Source: three-view drawing plus pictorial views. Frame: mm from the lowest corner of the part. A direction names the side the tool comes from. Coordinates: 2 decimals unless noted, no trailing zeros. Write each loop counter-clockwise with the first axis right and the second up, starting at its lowest first coordinate (ties: lowest second). Pieces come first, ordered by that corner, then holes. Notation, with made-up numbers: (-27.5, -40) - (14.5, -40) arc R23 cw to (14.5, -13) - close; hole circle Ø2 at (10.5, 68.25). An arc over 180 degrees is marked (long way). One line per item, written item: value.
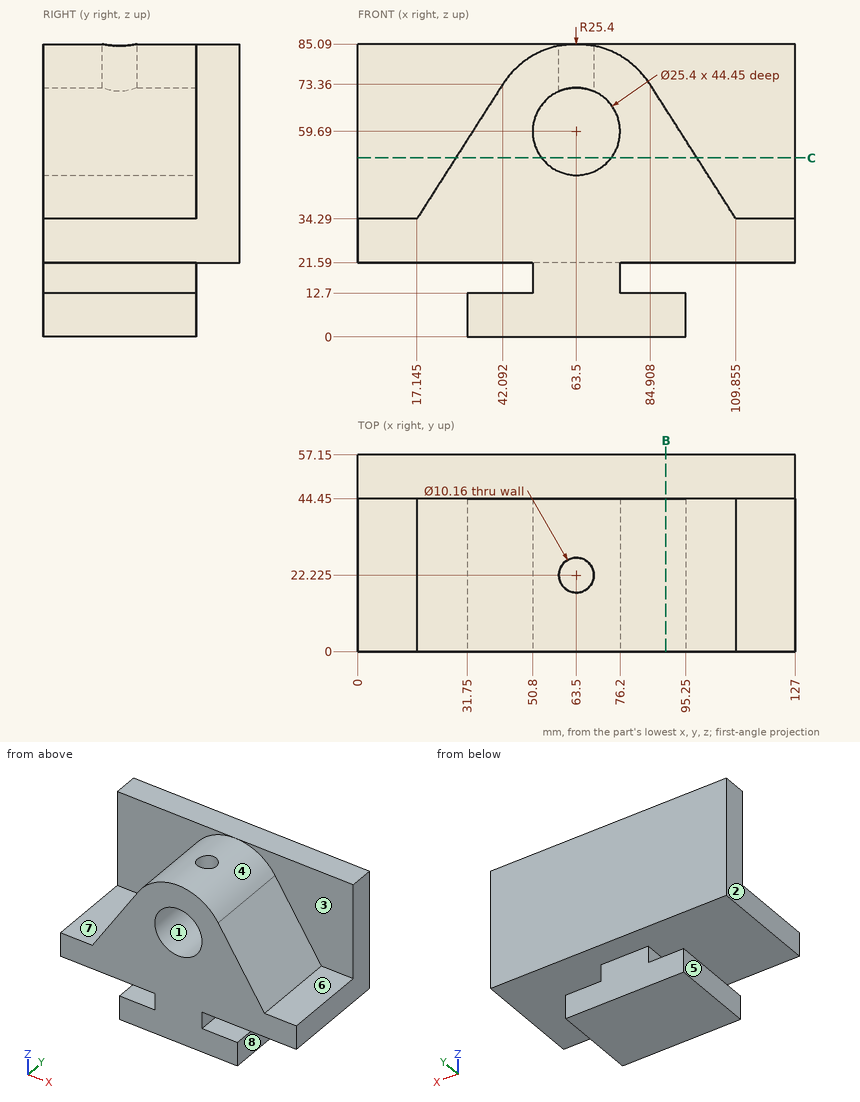
1) Section query C-C on z = 52. Output: boundary loops of the cut face in (x, y), then the cut area to 3 significant figures.
Values found:
outline: (0, 44.45) - (28.45, 44.45) - (28.45, 0) - (53.39, 0) - (53.39, 44.45) - (73.61, 44.45) - (73.61, 0) - (98.55, 0) - (98.55, 44.45) - (127, 44.45) - (127, 57.15) - (0, 57.15) - close
area: 3,830 mm2
2) Material intervals for line 1 (Z direction, x = 63.5, y = 10); line 2 (Z direction, x = 9.5, y = 5); line 3 (Y direction, x = 55, z = 19), sorted ascending.
Values found:
line 1: 0 to 46.99, 72.39 to 85.09
line 2: 21.59 to 34.29
line 3: 0 to 44.45
3) Contact query for flat-ended pins moving along their axis: P1, Ø19, axis at x = 12, y = 27, coming from the +Z side; P2, Ø7, axis at y = 27, z = 17.5, coming from the +X side; P3, Ø12.5, axis at x = 64.5, z = 60, coming from the -Y side. Output: stop coordinate, or through.
Values found:
P1: z = 41.11
P2: x = 76.2
P3: y = 44.45
4) Reachability of the marked faces 4, 5, 6, 7 and 8 from +Z, -Z, +X, -X, +Y, -Y: full face, straight path, thin tool, end or side. Return the list, or none.
Values found:
face 4: +Z, -Y
face 5: -Z, -X, +Y, -Y
face 6: +Z, +X, -Y
face 7: +Z, -X, -Y
face 8: -Z, +X, +Y, -Y
5) Draft query along X for the marked faces 1, 2 and 3. Return one class per face: released by +X, released by -X, zero draft, split by the parting line, or undercut.
Values found:
face 1: undercut
face 2: released by -X
face 3: zero draft
6) Section query B-B on x = 89.5. Output: boundary loops of the cut face in (y, z).
Values found:
outline: (0, 0) - (44.45, 0) - (44.45, 12.7) - (0, 12.7) - close; (0, 21.59) - (57.15, 21.59) - (57.15, 85.09) - (44.45, 85.09) - (44.45, 66.17) - (0, 66.17) - close
